Can you work these out from the model? Positions are in its coordinate system, mm. A direction names the side the tool comes from. Round coordinates to 2 decimals unless told otherwise and drop trailing zeros. Loops run counter-clockwise (first coordinate to the right, second up) from the corner with the lowest first, then second, coordinate; pieces in that order, holes last.
(1) Which directions (+Z, -Z, +X, -X, +Y, -Y) give clear straight access to the entire face, cutting with the end or side of a thin tool? Please do faces 1 (the face through (-12.7, 13, 0)), 2 (the face through (11, 13, 10.478)), 3 (the face through (10.795, 13, 12)), 4 (the face through (0, 0, 0)), 5 (the face through (10.16, 13, 1)).
(2) Will these pins go through, and if not, where does the flat tip stop? pin 1 Ø1.5 at (x, z) = (3.5, 8.5) entering from -Y; pin 2 Ø3 at (x, y) = (6.5, 10) entering from +Z.
(3) If I drill on line 1 along X through (y, z) = (4.25, 10.75) (3 decimals); line 2 along X through (y, z) = (20.75, -4.5); line 3 along Y through (x, z) = (-0.5, -5.25), over which ranges is the centre line in solid material (lowest first)?
(4) I want a section at A-A on y = 20.75. Write out the boundary of the cut face in (x, z) (1 decimal), plus the area to 3 significant figures.
(5) Thinking about a two-plate mould opening in Y: for faces 6 (the face through (0, 2.54, 1)), 7 (the face through (0, 13, -10.16)), 8 (the face through (0, 25.4, 0)), 9 (the face through (-10.795, 13, 12)), which applies, released by +Y, released by -Y, zero draft, split by the parting line, or undercut?
(6) I want a section at C-C on x = 7.25. Write out the boundary of the cut face in (y, z).
(7) I want a section at B-B on z = 6. Write out the boundary of the cut face in (x, y), plus the area to 3 significant figures.
from build123d import *

# Parameters (mm, degrees)
F2_DEPTH = 11.43
F3_DEPTH = 25.4
F4_T     = -2.54
F7_DEPTH = 25.4


with BuildPart() as f2:
    # F1 (on Top) → F2 (new body, symmetric)
    with BuildSketch(Plane.XY):
        Polygon((0, 1.27), (11.43, 1.27), (11.43, 24.13), (-11.43, 24.13), (-11.43, 1.27), align=None)
    extrude(amount=F2_DEPTH, both=True)


with BuildPart() as f3:
    # F0 (on Front) → F3 (new body)
    with BuildSketch(Plane.XZ):
        Polygon((-12.7, -12.7), (12.7, -12.7), (12.7, 12.7), (0, 12.7), (-12.7, 12.7), align=None)
    extrude(amount=-F3_DEPTH)

    # F4
    f4_openings = [f3.faces().sort_by_distance(p)[0] for p in [
        (0, 12.7, 12.7),
    ]]
    offset(amount=F4_T, openings=f4_openings)

    # F6 (on Front) → F7 (cut)
    with BuildSketch(Plane.XZ):
        Polygon((-12.065, 10.4775), (-10.795, 10.4775), (-10.795, 11.1125), (-10.795, 12.7), (-11.684, 12.7), (-11.684, 11.90625), (-12.065, 11.1125), align=None)
        Polygon((10.795, 10.4775), (12.065, 10.4775), (12.065, 11.1125), (11.684, 11.90625), (11.684, 12.7), (10.795, 12.7), (10.795, 11.1125), align=None)
    extrude(amount=-F7_DEPTH, mode=Mode.SUBTRACT)


solid = f3.part
Filled sheet:
1. face 1: +Z, -Z, -X, +Y, -Y
1. face 2: +Y, -Y
1. face 3: +Z, +Y, -Y
1. face 4: +Z, -Z, +X, -X, -Y
1. face 5: +Z
2. pin 1: stops at y = 0
2. pin 2: stops at z = -10.16
3. line 1: x = -12.7 to -12.065, -10.795 to -10.16, 10.16 to 10.795, 12.065 to 12.7
3. line 2: x = -12.7 to -10.16, 10.16 to 12.7
3. line 3: y = 0 to 2.54, 22.86 to 25.4
4. outline: (-12.7, -12.7) - (12.7, -12.7) - (12.7, 12.7) - (11.7, 12.7) - (11.7, 11.9) - (12.1, 11.1) - (12.1, 10.5) - (10.8, 10.5) - (10.8, 12.7) - (10.2, 12.7) - (10.2, -10.2) - (-10.2, -10.2) - (-10.2, 12.7) - (-10.8, 12.7) - (-10.8, 10.5) - (-12.1, 10.5) - (-12.1, 11.1) - (-11.7, 11.9) - (-11.7, 12.7) - (-12.7, 12.7) - close
4. area: 176 mm2
5. face 6: undercut
5. face 7: undercut
5. face 8: released by +Y
5. face 9: zero draft
6. outline: (0, -12.7) - (25.4, -12.7) - (25.4, 12.7) - (22.86, 12.7) - (22.86, -10.16) - (2.54, -10.16) - (2.54, 12.7) - (0, 12.7) - close
7. outline: (-12.7, 0) - (12.7, 0) - (12.7, 25.4) - (-12.7, 25.4) - close; hole (-10.16, 2.54) - (10.16, 2.54) - (10.16, 22.86) - (-10.16, 22.86) - close
7. area: 232 mm2
